Autodesk Inventor part; units mm, degrees
ref_plane "YZ Plane" through (0, 0, 0) normal (1, 0, 0) x (0, 1, 0)
ref_plane "XZ Plane" through (0, 0, 0) normal (0, 1, 0) x (-1, 0, 0)
ref_plane "XY Plane" through (0, 0, 0) normal (0, 0, 1) x (1, 0, 0)
sketch "Sketch1" plane through (0, 0, 0) normal (0, 1, 0) x (-1, 0, 0)
  line L0 (25, 34) -> (-25, 34)
  line L1 (-25, 34) -> (-25, -34)
  line L2 (-25, -34) -> (25, -34)
  line L3 (25, -34) -> (25, 34)
  line L4 (25, 34) -> (-25, -34) construction
  line L5 (-25, 34) -> (25, -34) construction
  point P0 (0, 0)
  dimension "d0" = 68
  dimension "d1" = 50
extrude "left wall" add sketch "Sketch1" along normal blind 2
sketch "Sketch3" plane through (0, 2, 0) normal (0, 1, 0) x (1, 0, 0)
  line L0 (25, -34) -> (25, 34)
  line L1 (-25, 34) -> (-25, -34)
  line L2 (25, -34) -> (-25, -34)
  line L3 (-25, -34) -> (-25, -32)
  line L4 (-25, -32) -> (25, -32)
  line L5 (25, -32) -> (25, -34)
  point P0 (0, 0)
  dimension "d4" = 2
extrude "bottom wall" add sketch "Sketch3" along normal blind 110.9
sketch "Sketch10" plane through (-25, 2, 32) normal (0, 0, -1) x (-1, 0, 0)
  line L0 (0, 0) -> (0, 110.9)
  line L1 (-50, 0) -> (-50, 110.9)
  line L2 (0, 58.9) -> (-50, 58.9)
  line L3 (-50, 58.9) -> (-50, 61.9)
  line L4 (-50, 61.9) -> (0, 61.9)
  line L5 (0, 61.9) -> (0, 58.9)
  line L6 (-50, 0) -> (0, 0)
  point P0 (-25, -2)
  point P1 (0, 61.9)
  point P2 (-50, 58.9)
  dimension "d33" = 3
  dimension "d34" = 58.9
extrude "mid wall" add sketch "Sketch10" along normal blind 48 contours L2 L1 L4 L0
sketch "Sketch11" plane through (-25, 60.9, 32) normal (0, -1, 0) x (1, 0, 0)
  circle A0 centre (24, -24) radius 2.9
  line L0 (0, 0) -> (0, -48)
  line L1 (0, -48) -> (50, -48)
  dimension "d37" = 5.8
  dimension "d136" = 24
  dimension "d137" = 24
extrude "middle bearing hole" cut sketch "Sketch11" against normal blind 48
sketch "Sketch15" plane through (0, 2, 0) normal (0, 1, 0) x (1, 0, 0)
  line L0 (25, 34) -> (-25, 34)
  line L1 (-25, -32) -> (25, -32)
  line L2 (25, 34) -> (23, 34)
  line L3 (23, 34) -> (23, -32)
  line L4 (23, -32) -> (25, -32)
  line L5 (25, -32) -> (25, 34)
  point P0 (0, 0)
  point P1 (25, -32)
  dimension "d69" = 2
extrude "back wall" add sketch "Sketch15" along normal blind 110.9
sketch "Sketch20" plane through (-25, 60.9, -16) normal (0, -1, 0) x (1, 0, 0)
  circle A0 centre (24, 24) radius 4
  line L0 (0, 48) -> (48, 48)
  line L1 (48, -18) -> (0, -18)
  line L2 (0, -18) -> (0, 48)
  line L3 (0, 48) -> (48, 48)
  line L4 (48, 48) -> (48, -18)
  line L5 (0, 0) -> (48, 0)
  point P0 (25, 16)
  point P1 (48, 48)
  point P2 (24, 0)
  dimension "d106" = 8
  dimension "d138" = 24
  dimension "d139" = 24
extrude "thicker mid wall ring for bearing" cut sketch "Sketch20" against normal blind 0.5
sketch "Sketch21" plane through (23, 2, 32) normal (0, 0, -1) x (-1, 0, 0)
  line L0 (0, 0) -> (0, 59.4)
  line L1 (48, -2) -> (48, 110.9)
  line L2 (0, 45) -> (48, 45)
  line L3 (48, 45) -> (48, 47.9)
  line L4 (48, 47.9) -> (0, 47.9)
  line L5 (0, 47.9) -> (0, 45)
  line L6 (0, 0) -> (48, 0)
  point P0 (23, -2)
  dimension "d110" = 45
  dimension "d111" = 2.9
extrude "motor attachment wall" add sketch "Sketch21" along normal up to surface (66 mm away) contours L0 L4 L1 L2
sketch "Sketch24" plane through (-25, 47, 32) normal (0, -1, 0) x (1, 0, 0)
  circle A0 centre (24, -24) radius 2.95
  circle A1 centre (20.818, -20.818) radius 0.8
  circle A2 centre (27.182, -27.182) radius 0.8
  line L0 (48, -66) -> (48, 0)
  line L1 (0, 0) -> (0, -66)
  line L2 (48, 0) -> (0, 0)
  line L3 (0, 0) -> (0, -48)
  line L4 (0, -48) -> (48, -48)
  line L5 (48, -48) -> (48, 0)
  line L6 (48, -48) -> (0, 0)
  point P0 (25, 14.5)
  dimension "d119" = 5.9
  dimension "d125" = 48
  dimension "d126" = 62.5
  dimension "d127" = 24
  dimension "d128" = 24
  dimension "d131" = 1.6
  dimension "d132" = 4.5
  dimension "d133" = 4.5
extrude "motor holes" cut sketch "Sketch24" against normal up to surface (2.9 mm away) contours A0 L6 | L6 A0 | L6 A1 | A1 L6 | L6 A2 | A2 L6
sketch "Sketch25" plane through (-25, 47, 32) normal (0, -1, 0) x (1, 0, 0)
  line L0 (48, -48) -> (0, 0)
  line L1 (0, 0) -> (0, -66)
  line L2 (0, 0) -> (0, -66)
  line L3 (48, -66) -> (0, -66)
  circle A0 centre (24, -24) radius 2.95
  circle A1 centre (24, -24) radius 9
  line L4 (48, -48) -> (0, -48)
  line L5 (48, -48) -> (48, -66)
  line L6 (50, 2) -> (50, -66)
  line L7 (0, 0) -> (0, 2)
  line L8 (0, -66) -> (0, 0)
  point P0 (25, -32)
  point P1 (30.364, -30.364)
  point P2 (17.636, -17.636)
  dimension "d134" = 18
extrude "motor attachment wall cut out" cut sketch "Sketch25" against normal blind 3.075 contours L4 L1 L0 A1 | L5 L3 L1 L4
sketch "Sketch26" plane through (-25, 61.4, -16) normal (0, -1, 0) x (1, 0, 0)
  line L0 (48, 0) -> (0, 48)
  circle A0 centre (24, 24) radius 4
  circle A1 centre (24, 24) radius 2.9
  line L1 (0, 0) -> (48, 0)
  line L2 (48, 0) -> (0, 0)
  line L3 (0, 48) -> (0, 50)
  line L4 (0, 0) -> (0, 48)
  line L5 (24, 24) -> (48, 24)
  line L6 (48, 48) -> (48, 0)
  line L7 (24, 24) -> (24, 48)
  line L8 (48, 48) -> (0, 48)
  line L9 (21.1716, 26.8284) -> (24, 29.6569)
  line L10 (26.8284, 21.1716) -> (29.6569, 24)
  point P0 (25, -38)
  point P1 (24, 28)
  dimension "d140" = 8
extrude "mid wall cut out" cut sketch "Sketch26" against normal blind 3.075 contours L1 L4 L0 A0 | L0 L10 L5 L6 | L0 L8 L7 L9
sketch "Sketch27" plane through (23, 112.9, 32) normal (0, 0, -1) x (-1, 0, 0)
  line L0 (0, 0) -> (0, -49)
  line L1 (48, -112.9) -> (48, 0)
  line L2 (0, -27) -> (48, -27)
  line L3 (48, -27) -> (48, -25)
  line L4 (48, -25) -> (0, -25)
  line L5 (0, -25) -> (0, -27)
  line L6 (0, -110.9) -> (48, -110.9)
  point P0 (23, -112.9)
  point P1 (0, -25)
  dimension "d144" = 83.9
  dimension "d145" = 2
extrude "encoder wall" add sketch "Sketch27" along normal blind 48
sketch "Sketch28" plane through (-25, 85.9, 32) normal (0, -1, 0) x (1, 0, 0)
  line L0 (48, -48) -> (48, 0)
  line L1 (0, 0) -> (0, 2)
  line L2 (48, -48) -> (0, 0)
  circle A0 centre (24, -24) radius 3
  circle A1 centre (30.0104, -30.0104) radius 1.4
  circle A2 centre (17.9896, -17.9896) radius 1.4
  dimension "d153" = 6
  dimension "d154" = 8.5
  dimension "d155" = 8.5
  dimension "d156" = 2.8
  dimension "d157" = 2.8
extrude "encoder holes" cut sketch "Sketch28" against normal blind 48
sketch "Sketch29" plane through (-25, 85.9, 32) normal (0, -1, 0) x (1, 0, 0)
  line L0 (0, -48) -> (48, -48)
  line L1 (48, 0) -> (0, 0)
  line L2 (48, -48) -> (0, 0)
  circle A0 centre (24, -24) radius 11
  line L3 (0, 0) -> (0, 2)
  line L4 (0, 0) -> (0, -48)
  line L5 (0, -48) -> (48, -48)
  point P0 (25, -32)
  point P1 (31.7782, -31.7782)
  point P2 (16.2218, -16.2218)
  dimension "d160" = 22
extrude "encoder wall cut out" cut sketch "Sketch29" against normal blind 48 contours L4 L2 A0 L0
sketch "Sketch30" plane through (25, 0, -34) normal (0, 0, -1) x (-1, 0, 0)
  line L0 (2, 112.9) -> (50, 112.9)
  line L1 (50, 0) -> (0, 0)
  line L2 (50, 112.9) -> (0, 112.9)
  line L3 (0, 112.9) -> (0, 0)
  line L4 (0, 0) -> (50, 0)
  line L5 (50, 0) -> (50, 112.9)
  point P0 (25, 0)
extrude "top" add sketch "Sketch30" along normal blind 2
sketch "Sketch31" plane through (25, 0, -34) normal (0, 0, 1) x (1, 0, 0)
  point P0 (-25, 0)
sketch "Sketch32" plane through (25, 0, -34) normal (0, 0, 1) x (1, 0, 0)
  line L0 (-50, 0) -> (-50, 112.9)
  line L1 (0, 112.9) -> (0, 0)
  line L2 (-50, 111.9) -> (-1, 111.9)
  line L3 (-1, 111.9) -> (-1, 109.9)
  line L4 (-1, 109.9) -> (-50, 109.9)
  line L5 (-50, 109.9) -> (-50, 111.9)
  line L6 (-50, 112.9) -> (0, 112.9)
  point P0 (-25, 0)
  point P1 (0, 112.9)
  dimension "d165" = 1
  dimension "d166" = 2
  dimension "d177" = 1
extrude "top rightWallGroove" cut sketch "Sketch32" against normal blind 1
sketch "Sketch33" plane through (23, 2, 32) normal (-1, 0, 0) x (0, 0, 1)
  line L0 (-78, 107.9) -> (-78, 104.9)
  line L1 (0, 110.9) -> (0, 85.9)
  line L2 (-78, 107.9) -> (0, 107.9)
  line L3 (0, 107.9) -> (0, 109.9)
  line L4 (0, 109.9) -> (-78, 109.9)
  line L5 (-78, 109.9) -> (-78, 107.9)
  line L6 (-66, 110.9) -> (0, 110.9)
  point P0 (-32, -2)
  point P1 (-78, 109.9)
  point P2 (0, 107.9)
  dimension "d169" = 2
  dimension "d178" = 1
extrude "back rightWallGroove" cut sketch "Sketch33" against normal blind 1
sketch "Sketch34" plane through (23, 112.9, 32) normal (0, 0, -1) x (-1, 0, 0)
  line L0 (48, -112.9) -> (48, 0)
  line L1 (48, -3) -> (-1, -3)
  line L2 (-1, -3) -> (-1, -1)
  line L3 (-1, -1) -> (48, -1)
  line L4 (48, -1) -> (48, -3)
  line L5 (48, 0) -> (-2, 0)
  line L6 (-2, -112.9) -> (-2, 0)
  point P0 (23, -112.9)
  point P1 (-1, -2)
  point P2 (48, -1)
  dimension "d172" = 1
  dimension "d173" = 2
  dimension "d174" = 1
extrude "bottom rightWallGroove" cut sketch "Sketch34" against normal blind 1
sketch "Sketch35" plane through (-25, 85.9, 32) normal (0, -1, 0) x (1, 0, 0)
  circle A0 centre (24, -24) radius 3
  circle A1 centre (24, -24) radius 3
  circle A2 centre (24, -24) radius 5
  point P0 (25, -32)
  dimension "d179" = 2
extrude "encoder bearing thicker" add sketch "Sketch35" along normal blind 1
ref_plane "Work Plane4" through (-1, 72.9, 32) normal (0, 1, 0) x (1, 0, 0)
sketch "Sketch38" plane through (23, 2, 32) normal (-1, 0, 0) x (0, 0, 1)
  line L0 (-66, 0) -> (-66, 107.9)
  line L1 (-66, 70.9) -> (-23.3371, 70.9)
  line L2 (-66, 0) -> (0, 0)
  line L3 (-56, 0) -> (-56, 123.7656)
  line L4 (-48, 45) -> (-48, 47.9)
  line L5 (-82, 70.9) -> (16, 70.9)
  line L6 (-62, 18.53) -> (-50, 18.53)
  line L7 (-50, 18.53) -> (-50, 25.53)
  line L8 (-50, 25.53) -> (-62, 25.53)
  line L9 (-62, 25.53) -> (-62, 18.53)
  line L10 (-62, 18.53) -> (-50, 25.53) construction
  line L11 (-50, 18.53) -> (-62, 25.53) construction
  circle A0 centre (-56, 70.9) radius 1.5
  point P0 (-32, -2)
  point P1 (-48, 46.45)
  point P2 (-56, 22.03)
  dimension "d195" = 8
  dimension "d196" = 0
  dimension "d197" = 7
  dimension "d198" = 12
  dimension "d199" = 52.37
  dimension "d202" = 3
extrude "loadcell block" add sketch "Sketch38" along normal blind 30 contours L6 L9 L8 L3 | L3 L8 L7 L6
extrude "wire exit" cut sketch "Sketch38" against normal blind 30 contours A0 L3 L1 | L1 L3 A0 | L3 A0 L1 | L1 A0 L3
sketch "Sketch39" plane through (-7, 2, 32) normal (-1, 0, 0) x (0, 0, 1)
  line L0 (-50, 25.53) -> (-50, 18.53)
  line L1 (-50, 22.03) -> (-62, 22.03)
  line L2 (-62, 25.53) -> (-62, 18.53)
  line L3 (-62, 18.53) -> (-50, 18.53)
  line L4 (-50, 18.53) -> (-62, 18.53)
  line L5 (-56, 18.53) -> (-56, 25.53)
  line L6 (-62, 25.53) -> (-50, 25.53)
  circle A0 centre (-59, 22.03) radius 1.5
  circle A1 centre (-53, 22.03) radius 1.5
  point P0 (-32, -2)
  dimension "d205" = 3.5
  dimension "d206" = 6
  dimension "d207" = 6
  dimension "d208" = 3
  dimension "d209" = 3
extrude "loadcell screw holes" cut sketch "Sketch39" against normal blind 10 contours A1 L1 | L1 A1 | A0 L1 | L1 A0
sketch "Sketch40" plane through (23, 27.53, -18) normal (0, 1, 0) x (1, 0, 0)
  line L0 (0, -52) -> (0, 16)
  line L1 (0, 10) -> (-16, 10)
  line L2 (-16, 10) -> (-16, 2)
  line L3 (-16, 2) -> (0, 2)
  line L4 (0, 2) -> (0, 10)
  line L5 (-30, 0) -> (-30, 12)
  line L6 (0, 0) -> (-30, 0)
  line L7 (0, 12) -> (-30, 12)
  point P0 (-23, -18)
  point P1 (-16, 6)
  point P2 (-30, 6)
  point P3 (0, 2)
  dimension "d215" = 14
  dimension "d216" = 2
  dimension "d217" = 2
extrude "Extrusion32" cut sketch "Sketch40" against normal blind 10 contours L3 L2 L1 L0
fillet "Fillet1" radius 2 4 edges at (7, 24.03, -28) (7, 24.03, -20) (23, 24.03, -20) (23, 24.03, -28)
fillet "Fillet2" radius 1 2 edges at (23, 72.9, -25.5) (25, 72.9, -25.5)
sketch "Sketch41" plane through (23, 20.53, -30) normal (0, 0, -1) x (-1, 0, 0)
  line L0 (0, 0) -> (30, 0)
  line L1 (0, 7) -> (30, 7)
  line L2 (30, 0) -> (23, 0)
  line L3 (23, 0) -> (23, 7)
  line L4 (23, 7) -> (30, 7)
  line L5 (30, 7) -> (30, 0)
  point P0 (23, -20.53)
  point P1 (23, 3.5)
  point P2 (23, 0)
  dimension "d225" = 7
extrude "load cell block support" add sketch "Sketch41" along normal up to surface (4 mm away)
equation "\"d136\" = d127"
equation "\"d137\" = d136"
equation "\"d69\" = d4"
equation "\"d70\" = d5"
equation "\"d139\" = d138"
equation "\"d127\" = 0.5 * d125"
equation "\"d128\" = d127"
equation "\"d133\" = d132"
equation "\"d134\" = 4 * d132"
equation "\"d140\" = d106"
equation "\"d146\" = d125"
properties part number "motor_maincase1.1_3DPrint"
The model under review builds one solid part; all positions refer to its coordinate system, in mm. A direction names the side the tool comes from. Coordinates: 2 decimals unless noted, no trailing zeros. Write each loop counter-clockwise with the first axis right and the second up, starting at its lowest first coordinate (ties: lowest second). Pieces come first, ordered by that corner, then holes. Notation, with made-up numbers: (26, -17) - (51, -17) arc R29 cw to (51, 20) - close; hole circle Ø9 at (44, -7.75). An arc over 180 degrees is marked (long way). Answer in a Markdown table with one row per item. Add a question column.
Q1. Consider section C-C on y = 37.5. Give the boundary of the cut face in (x, z).
Q2. Consider section B-B on y = 24.03. Give the number of separate pieces and of enclosed holes in the cut face, then the cut area to 3 significant figures.
Q3. Clearance check with flat-ended pins moving along their axes: pin 1 (7 mm diameter, centred on x = -1, z = 8, fed in from +Y); pin 2 (14.5 mm diameter, centred on x = -7, z = -11, fed in from +Y); pin 3 (20 mm diameter, centred on y = 50, z = -12.5, fed in from -X). State where each tip first meets the part, or that it passes through.
Q4. For faces 4 (the face through (3.223, 62.632, 6.566)), 5 (the face through (-1, 99, 32)), 6 (the face through (2, 20.53, -24)), list the 3-axis set-ups (+Z, -Z, +X, -X, +Y, -Y) from which the entire face can be reached by the end or side of a thin tool; tool diameter is ignored.
Q5. Draft analysis for pull direction Y (two halves, no side actions). For faces 1 (the face through (3, 24, -21)), 2 (the face through (24, 112.9, -1)), 3 (the face through (8, 24, -18)), state which applies: +Y half, -Y half, draft (parallel to the pull), parting line (faces both ways), or undercut.
Q6. To check wall thickness, follow line 1 along Y through (x, z) = (-6, 25.5); line 2 along Y through (x, z) = (19.5, 25); line 3 along Z through (x, y) = (2, 18.5). State the ranges of each line that lie inside material, in increasing order. Write a range as from..to.
Q7. Consider section A-A on z = 28. Give the boundary of the cut face in (x, y).
Answers below:
| question | item | result |
|---|---|---|
| 1 | outline | (-25, -36) - (25, -36) - (25, 34) - (-25, 34) - (-25, 32) - (23, 32) - (23, -34) - (-25, -34) - close |
| 2 | separate pieces | 1 |
| 2 | enclosed holes | 2 |
| 2 | area | 535 mm² |
| 3 | pin 1 | y = 87.9 |
| 3 | pin 2 | y = 27.53 |
| 3 | pin 3 | x = 9.5 |
| 4 | face 4 | none |
| 4 | face 5 | -X, +Y |
| 4 | face 6 | -X |
| 5 | face 1 | undercut |
| 5 | face 2 | +Y half |
| 5 | face 3 | draft |
| 6 | line 1 | 0..2, 47..49.9, 85.9..87.9 |
| 6 | line 2 | 0..2, 47..49.9, 61.4..63.9, 85.9..87.9 |
| 6 | line 3 | -36..-34, 32..34 |
| 7 | outline | (-25, 0) - (25, 0) - (25, 112.9) - (23, 112.9) - (23, 111.9) - (24, 111.9) - (24, 109.9) - (23, 109.9) - (23, 87.9) - (-21, 87.9) - (-21, 85.9) - (23, 85.9) - (23, 63.9) - (-1, 63.9) - (-1, 61.4) - (23, 61.4) - (23, 49.9) - (-21, 49.9) - (-21, 47) - (23, 47) - (23, 2) - (-25, 2) - close |
